Part model, mm, in its own coordinate system. A direction names the side the tool comes from. Round coordinates to 2 decimals unless told otherwise and drop trailing zeros. Write each loop counter-clockwise with the first axis right and the second up, starting at its lowest first coordinate (ties: lowest second). Pieces come first, ordered by that corner, then holes. Notation, with made-up numbers: (57, 17) -> (69, 17) arc R32 ccw to (69, 49) -> close; hole circle Ø8 at (-14, 18). An arc over 180 degrees is marked (long way). Use CSV: the item, a comma, the result in double quotes. Start each with the question number.
```python
from build123d import *

# Parameters (mm, degrees)
EXTRUDE_1_DEPTH     = 2
SKETCH_2_R          = 6
EXTRUDE_2_DEPTH     = 10
SKETCH_3_R          = 5
CUT_EXTRUDE_1_DEPTH = 5


with BuildPart() as part:
    # ｽｹｯﾁ1 → ﾎﾞｽ - 押し出し1 (new body)
    with BuildSketch(Plane(origin=(0, 0, 0), x_dir=(1, 0, 0), z_dir=(0, 1, 0))):
        Polygon((4.062937169, -6.987551424), (8.082865627, 0.02483109), (4.019928459, 7.012382514), (-4.062937169, 6.987551424), (-8.082865627, -0.02483109), (-4.019928459, -7.012382514), align=None)
    extrude(amount=EXTRUDE_1_DEPTH)

    # ｽｹｯﾁ2 → ﾎﾞｽ - 押し出し2 (add)
    with BuildSketch(Plane(origin=(0, 2, 0), x_dir=(1, 0, 0), z_dir=(0, 1, 0))):
        with Locations(Location((0, 0, 0), (0, 0, 270))):
            Circle(SKETCH_2_R)
    extrude(amount=EXTRUDE_2_DEPTH)

    # ｽｹｯﾁ3 → ｶｯﾄ - 押し出し1 (cut)
    with BuildSketch(Plane(origin=(0, 12, 0), x_dir=(1, 0, 0), z_dir=(0, 1, 0))):
        with Locations(Location((0, 0, 0), (0, 0, 270))):
            Circle(SKETCH_3_R)
    extrude(amount=-CUT_EXTRUDE_1_DEPTH, mode=Mode.SUBTRACT)


solid = part.part
```
1. Band-saw the part on B-B (z = -1.75). List the corners of the cut face in (x, y), then the cut area to 3 significant figures.
2. Which spindle directions (+Z, -Z, +X, -X, +Y, -Y) get a long thin tool onto all of the face, cutting with end or side? Do faces 1 (the cylindrical face through (-4.88, 9.54, -1.08)), 2 (the flat face through (0, 0, 0)). Say none if no direction does.
3. Band-saw the part on D-D (y = 5.5). List the corners of the cut face in (x, z).
4. Band-saw the part on C-C (y = 11.25). List the corners of the cut face in (x, z), then the cut area to 3 significant figures.
5. Drill centre lines: line 1 along X through (y, z) = (8.7, 0); line 2 along Y through (x, z) = (1.25, 2.75); line 3 along Z through (x, y) = (4, 11.5). Where is each one in solid material? Low to high. Write a range as [from, to].
6. Pull direction X, two halves, no side cores. Call faces 3 (the flat face through (0, 7, 0)), 4 (the flat face through (6.045, 0.986, 3.53)), 5 (the cylindrical face through (1.802, 6.93, 5.723)), 6 (the flat face through (4, 12, -4)): released by +X, released by -X, zero draft, split by the parting line, or undercut.
7. Band-saw the part on A-A (x = -2). List the corners of the cut face in (y, z), then the cut area to 3 significant figures.
8. Flat gauge pins, fed straight in: pin 1 (3 mm diameter, centred on x = -4.5, z = -3, fed in from -Y); pin 2 (3 mm diameter, centred on y = 7.5, z = -3.5, fed in from +X); pin 3 (5 mm diameter, centred on x = -1, z = -0.5, fed in from +Y); pin 4 (4 mm diameter, centred on y = 10.5, z = 3.5, fed in from -X). Where does each tip first touch, or does it go through?
Answers below:
1,outline,"(-7.07, 0) -> (7.08, 0) -> (7.08, 2) -> (5.74, 2) -> (5.74, 12) -> (4.68, 12) -> (4.68, 7) -> (-4.68, 7) -> (-4.68, 12) -> (-5.74, 12) -> (-5.74, 2) -> (-7.07, 2) -> close"
1,area,"96.2 mm^2"
2,face 1,"+Y"
2,face 2,"+Z, -Z, +X, -X, -Y"
3,outline,"circle Ø12 at (0, 0)"
4,outline,"circle Ø12 at (0, 0); hole circle Ø10 at (0, 0)"
4,area,"34.6 mm^2"
5,line 1,"x = [-6, -5], [5, 6]"
5,line 2,"y = [0, 7]"
5,line 3,"z = [-4.47, -3], [3, 4.47]"
6,face 3,"undercut"
6,face 4,"released by +X"
6,face 5,"split by the parting line"
6,face 6,"zero draft"
7,outline,"(0, -6.99) -> (2, -6.99) -> (2, -5.66) -> (12, -5.66) -> (12, -4.58) -> (7, -4.58) -> (7, 4.58) -> (12, 4.58) -> (12, 5.66) -> (2, 5.66) -> (2, 7.01) -> (0, 7.01) -> close"
7,area,"95.3 mm^2"
8,pin 1,"stops at y = 0"
8,pin 2,"stops at x = 5.66"
8,pin 3,"stops at y = 7"
8,pin 4,"stops at x = -5.81"
